Read the model definition and answer for the solid it produces. Units are mm, in the model's axes. A direction names the side the tool comes from. Coordinates: 2 decimals unless noted, no trailing zeros. Loops run counter-clockwise (first coordinate to the right, second up) from the corner with the lowest first, then second, coordinate; pieces in that order, holes last. Notation, with made-up numbers: (-32, 29.25) -> (-6, 29.25) arc R20 ccw to (-6, 45.25) -> close; hole circle Ø9 at (-6, 15). An arc over 180 degrees is marked (long way). Answer in a Markdown table with one row per item.
```python
from build123d import *

# Parameters (mm, degrees)
F0_R     = 26
F0_R_2   = 22.5
F1_DEPTH = 15
F3_R     = 5.044876
F4_DEPTH = 11
F0_R_3   = 15.5
F0_R_4   = 12.5
F5_DEPTH = 15


with BuildPart() as f1:
    # F0 (on Front) → F1 (new body)
    with BuildSketch(Plane.XZ):
        Circle(F0_R)
        Circle(F0_R_2, mode=Mode.SUBTRACT)
    extrude(amount=-F1_DEPTH)

    # F3 (on offset) → F4 (join)
    with BuildSketch(Plane.XZ.offset(-2)):
        with Locations((0, -19.415323)):
            Circle(F3_R)
        with Locations((11.41204, -15.707326)):
            Circle(F3_R)
        with Locations((18.465069, -5.999665)):
            Circle(F3_R)
        with Locations((18.465069, 5.999665)):
            Circle(F3_R)
        with Locations((11.41204, 15.707326)):
            Circle(F3_R)
        with Locations((0, 19.415323)):
            Circle(F3_R)
        with Locations((-11.41204, 15.707326)):
            Circle(F3_R)
        with Locations((-18.465069, 5.999665)):
            Circle(F3_R)
        with Locations((-18.465069, -5.999665)):
            Circle(F3_R)
        with Locations((-11.41204, -15.707326)):
            Circle(F3_R)
    extrude(amount=-F4_DEPTH)

    # F0 (on Front) → F5 (join)
    with BuildSketch(Plane.XZ):
        Circle(F0_R_3)
        Circle(F0_R_4, mode=Mode.SUBTRACT)
    extrude(amount=-F5_DEPTH)


solid = f1.part
```
1. Find the intervals of material crossed by probe 1 along Z at (x, y) = (0, 5.5); probe 2 along Z at (x, y) = (10, 13.5); probe 3 along X at (y, z) = (6.5, -0.5), in increasing order.
A:
| item | result |
|---|---|
| probe 1 | z = -26 to -12.5, 12.5 to 26 |
| probe 2 | z = -24 to -20.16, -11.84 to -7.5, 7.5 to 11.84, 20.16 to 24 |
| probe 3 | x = -26 to -22.49, -15.49 to -12.49, 12.49 to 15.49, 22.49 to 26 |
2. Given pin 1 Ø9.5 at (x, z) = (19, -8) entering from +Y; pin 2 Ø2 at (x, y) = (12, 8.5) entering from +Z; pin 3 Ø1 at (y, z) = (12.5, -9.5) entering from +X; pin 4 Ø2.5 at (x, z) = (17.5, 3.5) entering from -Y, each flat-ended and moving along its own axis, determine where each tip first touches the part or whether it passes through.
A:
| item | result |
|---|---|
| pin 1 | stops at y = 15 |
| pin 2 | stops at z = 23.56 |
| pin 3 | stops at x = 24.39 |
| pin 4 | stops at y = 2 |
3. A cutting plane is placed at B-B on z = 0. Give the vertices of the cut face in (x, y), and give its area (3 significant figures).
A:
| item | result |
|---|---|
| outline | (-26, 0) -> (-22.5, 0) -> (-22.5, 15) -> (-26, 15) -> close; (-15.5, 0) -> (-12.5, 0) -> (-12.5, 15) -> (-15.5, 15) -> close; (12.5, 0) -> (15.5, 0) -> (15.5, 15) -> (12.5, 15) -> close; (22.5, 0) -> (26, 0) -> (26, 15) -> (22.5, 15) -> close |
| area | 195 mm2 |
4. A cutting plane is placed at D-D on y = 5.5. Count the separate pieces of the cut face and the enclosed holes in it, and give its area (3 significant figures).
A:
| item | result |
|---|---|
| separate pieces | 1 |
| enclosed holes | 11 |
| area | 1,430 mm2 |
5. A tool of negligible diameter and unlimited length cuts with its end or side. For faces 4 (the flat face through (0, 2, 19)), 5 (the flat face through (18, 13, -6)), 6 (the cylindrical face through (11.923, 7.395, 3.755)), from which of +Z, -Z, +X, -X, +Y, -Y can it reach the whole face along a straight path? Write none if from no direction.
A:
| item | result |
|---|---|
| face 4 | -Y |
| face 5 | +Y |
| face 6 | +Y, -Y |
6. A cutting plane is placed at C-C on x = 18.5. Give the vertices of the cut face in (y, z), and give its area (3 significant figures).
A:
| item | result |
|---|---|
| outline | (0, -18.27) -> (15, -18.27) -> (15, -12.81) -> (0, -12.81) -> close; (0, 12.81) -> (15, 12.81) -> (15, 18.27) -> (0, 18.27) -> close; (2, -11.04) -> (13, -11.04) -> (13, -0.95) -> (2, -0.95) -> close; (2, 0.95) -> (13, 0.95) -> (13, 11.04) -> (2, 11.04) -> close |
| area | 386 mm2 |
7. A cutting plane is placed at A-A on x = 0. Give the vertices of the cut face in (y, z), and give its area (3 significant figures).
A:
| item | result |
|---|---|
| outline | (0, -26) -> (15, -26) -> (15, -22.5) -> (13, -22.5) -> (13, -15.5) -> (15, -15.5) -> (15, -12.5) -> (0, -12.5) -> (0, -15.5) -> (2, -15.5) -> (2, -22.5) -> (0, -22.5) -> close; (0, 12.5) -> (15, 12.5) -> (15, 15.5) -> (13, 15.5) -> (13, 22.5) -> (15, 22.5) -> (15, 26) -> (0, 26) -> (0, 22.5) -> (2, 22.5) -> (2, 15.5) -> (0, 15.5) -> close |
| area | 349 mm2 |
8. The mould has two halves that part along Z. Classify faces 1 (the flat face through (-11.7, 15, 19.4)), 2 (the cylindrical face through (-20.633, 7.395, -15.821)), 3 (the cylindrical face through (-22.48, 7.4, 0.99)): pulls with the +Z half, pulls with the -Z half, needs draft (parallel to the pull), parting line crosses it, or undercut.
A:
| item | result |
|---|---|
| face 1 | needs draft |
| face 2 | parting line crosses it |
| face 3 | undercut |
